Geometry check sheet. Reference: the model listing, model coordinates, mm. A direction names the side the tool comes from. Round coordinates to 2 decimals unless told otherwise and drop trailing zeros. Loops run counter-clockwise (first coordinate to the right, second up) from the corner with the lowest first, then second, coordinate; pieces in that order, holes last. Notation, with made-up numbers: (21, -27) -> (75, -27) arc R8 cw to (75, -17) -> close; hole circle Ø9 at (87.25, -22.75). An arc over 180 degrees is marked (long way). Use a Markdown table: item, result. Add a question column.
Q1. Sectioned sample at B-B, the plane y = -4.25. Enter the section's corners in (x, z).
Q2. Set-up check for faces 1 (the face through (0, -25, 6)), 2 (the face through (-1, -10.2, 5.5)), 3 (the face through (-1.08, -26.83, -4.88)): record each of +Z, -Z, +X, -X, +Y, -Y from which the full face is reachable in a straight line by a thin tool's end or side.
Q3. Sectioned sample at C-C, the plane x = 4.5. Enter the section's corners in (y, z), then the cut area to 3 significant figures.
Q4. Release check for a two-part mould opening along Y. For faces 4 (the face through (-5.22, -24.65, -2.96)), 5 (the face through (0, 0, 0)), 6 (the face through (-1, -4.2, 5.5)) record: released by +Y, released by -Y, zero draft, split by the parting line, or undercut.
Q5. Gauge pin test, flat ends, axial feed: P1, Ø2, axis at y = -12, z = 4, coming from the -X side; P2, Ø3, axis at x = -2, z = 0, coming from the -Y side. Record the tip position at first contact, or that the pin passes through.
Q6. Sectioned sample at A-A, the plane y = -30. Enter the section's corners in (x, z), then the cut area to 3 significant figures.
Q7. Sectioned sample at D-D, the plane z = -0.75. Enter the section's corners in (x, y), then the cut area to 3 significant figures.
Q8. Material ranges on L1, parallel to Z at x = -0.25, y = -39.5; L2, parallel to Y at x = -0.5, z = 2.5; L3, parallel to X at y = -4.25, z = 5.35, recorded low to high.
```python
from build123d import *

# Parameters (mm, degrees)
F1_DEPTH = 50
F2_R     = 5
F3_DEPTH = 47
F4_R     = 1
F5_DEPTH = 2


with BuildPart() as f1:
    # F0 (on Front) → F1 (new body)
    with BuildSketch(Plane.XZ):
        Polygon((3.464102, 6), (-3.464102, 6), (-6.928203, 0), (-3.464102, -6), (3.464102, -6), (6.928203, 0), align=None)
    extrude(amount=F1_DEPTH)

    # F2 (on face) → F3 (cut)
    with BuildSketch(Plane.XZ.offset(50)):
        Circle(F2_R)
    extrude(amount=-F3_DEPTH, mode=Mode.SUBTRACT)

    # F4 (on face) → F5 (cut)
    with BuildSketch(Plane.XY.offset(6)):
        with Locations((0, -10.25)):
            Circle(F4_R)
        with Locations((0, -4.25)):
            Circle(F4_R)
    extrude(amount=-F5_DEPTH, mode=Mode.SUBTRACT)


solid = f1.part
```
Values:
| question | item | result |
|---|---|---|
| 1 | outline | (-6.93, 0) -> (-3.46, -6) -> (3.46, -6) -> (6.93, 0) -> (3.46, 6) -> (1, 6) -> (1, 4.9) arc R5 cw (long way) to (-1, 4.9) -> (-1, 6) -> (-3.46, 6) -> close |
| 2 | face 1 | +Z, +X, -X, +Y, -Y |
| 2 | face 2 | +Z |
| 2 | face 3 | -Y |
| 3 | outline | (-50, -4.21) -> (0, -4.21) -> (0, 4.21) -> (-50, 4.21) -> (-50, 2.18) -> (-3, 2.18) -> (-3, -2.18) -> (-50, -2.18) -> close |
| 3 | area | 216 mm^2 |
| 4 | face 4 | zero draft |
| 4 | face 5 | released by +Y |
| 4 | face 6 | undercut |
| 5 | P1 | x = -5.2 |
| 5 | P2 | y = -3 |
| 6 | outline | (-6.93, 0) -> (-3.46, -6) -> (3.46, -6) -> (6.93, 0) -> (3.46, 6) -> (-3.46, 6) -> close; hole circle Ø10 at (0, 0) |
| 6 | area | 46.2 mm^2 |
| 7 | outline | (-6.5, -50) -> (-4.94, -50) -> (-4.94, -3) -> (4.94, -3) -> (4.94, -50) -> (6.5, -50) -> (6.5, 0) -> (-6.5, 0) -> close |
| 7 | area | 185 mm^2 |
| 8 | L1 | -6 to -4.99, 4.99 to 6 |
| 8 | L2 | -3 to 0 |
| 8 | L3 | -3.84 to -1, 1 to 3.84 |
